Build history of the part. All positions in model axes, mm. Face numbers are marked on the shaded views. A direction names the side the tool comes from. Give positions to 0.01 mm unless a question says otherwise; leave off trailing zeros. Order: outer loops, then holes, each group sorted by start corner. A loop starts at its lowest first (then second) coordinate and runs counter-clockwise, first axis right, second up. Notation, with made-up numbers: M 42.5,-10 L 101.5,-10 A16 cw 101.5,8 Z; hole C -15.75,-22 d8. An arc over 180 degrees is marked long. Use CSV: the item, a comma, the result in double quotes. Start each with the question number.
Item 1: Band-saw the part on D-D on x = 3.75. Write the cut outline in (y, z).
Item 2: Pin check, flat tips, straight feed: P1, Ø1.1, axis at y = 5, z = -6, coming from the -X side; P2, Ø1.8, axis at y = 4, z = -4.5, coming from the +X side; P3, Ø0.9, axis at x = 5.5, y = 4.5, coming from the -Z side. Stop position of each tip, or through.
Item 3: Which spindle directions (+Z, -Z, +X, -X, +Y, -Y) get a long thin tool onto all of the face, cutting with end or side? Do the marked faces 1, 2, 3, 4 and 5. Say none if no direction does.
Item 4: Band-saw the part on B-B on z = -5.25. Write the cut outline in (x, y).
Item 5: Two-plate mould, pull along Y, no slides. Class the marked faces 6, 7, 8 and 9: pulls with the +Y half, pulls with the -Y half, needs draft (parallel to the pull), parting line crosses it, or undercut.
Item 6: Band-saw the part on C-C on z = 1.5. Write the cut outline in (x, y).
Item 7: Wall check: line 1 along X through (y, z) = (4, -3.5); line 2 along Y through (x, z) = (7.75, -0.5); line 3 along Z through (x, y) = (2.7, 4.4). Give the ranges that are in metal, low to high.
from build123d import *

# Parameters (mm, degrees)
F0_W         = 10.2
F0_H         = 7
F1_DEPTH     = 4
F2_W         = 6.2
F2_H         = 3.6
F3_DEPTH     = 7.2
F4_W         = 3
F4_H         = 4
F5_DEPTH     = 25
F6_R         = 1.79999
F7_R         = 1.1
F8_DEPTH     = 25
F9_R         = 3
F10_DEPTH    = 25
F11_T1_DEPTH = 17.2


# Not quite as in the source:
# - a fillet or chamfer that OpenCascade refuses, or shapes differently, is made with other operations: its cross-section is extruded or revolved along the edge and cut away or added
# - a fillet or chamfer is up to 0.001 mm smaller than in the source, because OpenCascade refuses the exact size


with BuildPart() as f1:
    # F0 (on Top) → F1 (new body)
    with BuildSketch(Plane.XY):
        with Locations((5.1, 3.5)):
            Rectangle(F0_W, F0_H)
    extrude(amount=F1_DEPTH)

    # F2 (on face) → F3 (join)
    with BuildSketch(Plane(origin=(0, 0, 0), x_dir=(1, 0, 0), z_dir=(0, 0, -1))):
        with Locations((5.1, -4.4)):
            Rectangle(F2_W, F2_H)
    extrude(amount=F3_DEPTH)

    # F4 (on face) → F5 (cut)
    with BuildSketch(Plane(origin=(0, 6.2, 0), x_dir=(-1, 0, 0), z_dir=(0, 1, 0))):
        with Locations((-5.1, -5.2)):
            Rectangle(F4_W, F4_H)
    extrude(amount=-F5_DEPTH, mode=Mode.SUBTRACT)

    # F6 (radius 1.8 in the source; OpenCascade refuses exactly that, so slightly less here)
    f6_edges = [f1.edges().sort_by_distance(p)[0] for p in [
        (2.8, 2.6, -7.2),
        (7.4, 2.6, -7.2),
        (2.8, 6.2, -7.2),
        (7.4, 6.2, -7.2),
    ]]
    fillet(f6_edges, radius=F6_R)

    # F7 (on face) → F8 (cut)
    with BuildSketch(Plane.YZ.offset(8.2)):
        with Locations((4.4, -5.4)):
            Circle(F7_R)
    extrude(amount=-F8_DEPTH, mode=Mode.SUBTRACT)

    # F9 (on face) → F10 (cut)
    with BuildSketch(Plane(origin=(0, 0, 0), x_dir=(0, -1, 0), z_dir=(-1, 0, 0))):
        with Locations((-2.6, 4)):
            Circle(F9_R)
    extrude(amount=-F10_DEPTH, mode=Mode.SUBTRACT)

    # F11: fillet of radius 2 on 1 edges, made by hand

    # F11_s2 → F11_t1 (cut)
    with BuildSketch(Plane.YZ.offset(-3.5)):
        with BuildLine():
            ThreePointArc((5.3518181818, 2.8052210689), (6.0125269518, 3.627994046), (7, 4))
            Line((7, 4), (5.6, 4))
            ThreePointArc((5.6, 4), (5.5372993162, 3.3898584367), (5.3518181818, 2.8052210689))
        make_face()
    extrude(amount=F11_T1_DEPTH, mode=Mode.SUBTRACT)


solid = f1.part
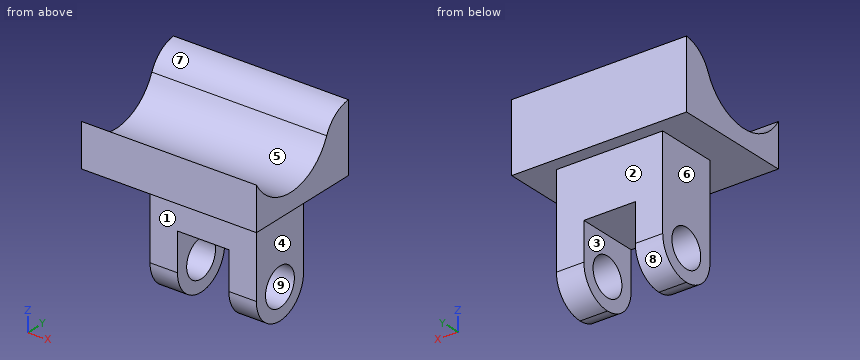
Model answer:
1,outline,"M 0,0 L 2.6,0 L 2.6,-3.2 L 6.2,-3.2 L 6.2,0 L 7,0 L 7,4 A2 ccw 5.35,2.81 A3 cw 0,2.5 Z"
2,P1,"stops at x = 2"
2,P2,"stops at x = 8.2"
2,P3,"stops at z = -3.2"
3,face 1,"-Z, +X, -X, -Y"
3,face 2,"-Z, +X, -X, +Y"
3,face 3,"-Z, +Y, -Y"
3,face 4,"-Z, +X, +Y, -Y"
3,face 5,"+Z, +X, -X"
4,outline,"M 2,2.6 L 3.6,2.6 L 3.6,3.31 L 2,3.31 Z; M 2,5.49 L 3.6,5.49 L 3.6,6.2 L 2,6.2 Z; M 6.6,2.6 L 8.2,2.6 L 8.2,3.31 L 6.6,3.31 Z; M 6.6,5.49 L 8.2,5.49 L 8.2,6.2 L 6.6,6.2 Z"
5,face 6,"needs draft"
5,face 7,"pulls with the -Y half"
5,face 8,"pulls with the +Y half"
5,face 9,"undercut"
6,outline,"M 0,0 L 10.2,0 L 10.2,0.94 L 0,0.94 Z; M 0,4.26 L 10.2,4.26 L 10.2,7 L 0,7 Z"
7,line 1,"x = 2 to 3.6, 6.6 to 8.2"
7,line 2,"y = 2.6 to 6.2"
7,line 3,"z = -7.2 to -6.5, -4.3 to 1.6"
